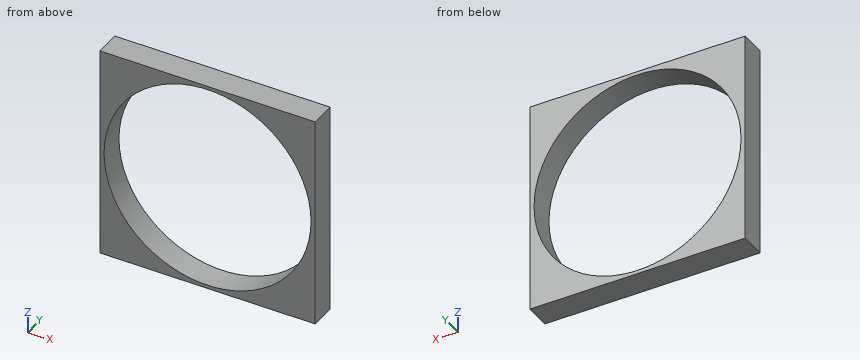
from build123d import *

# Parameters (mm, degrees)
F0_W     = 211.11551
F0_H     = 209.385068
F0_R     = 101.410764
F1_DEPTH = 25.4
F2_DEPTH = 25.4


with BuildPart() as f1:
    # F0 (on Front) → F1 (new body)
    with BuildSketch(Plane.XZ):
        Rectangle(F0_W, F0_H)
        Circle(F0_R, mode=Mode.SUBTRACT)
    extrude(amount=F1_DEPTH)

    # F0 (on Front) → F2 (join)
    with BuildSketch(Plane.XZ):
        Rectangle(F0_W, F0_H)
        Circle(F0_R, mode=Mode.SUBTRACT)
    extrude(amount=F2_DEPTH)


solid = f1.part
Design review of the part built by this model. Coordinates are the model's own, in mm. Give positions to 0.01 mm unless a question says otherwise; leave off trailing zeros. Order: outer loops, then holes, each group sorted by start corner. A loop starts at its lowest first (then second) coordinate and runs counter-clockwise, first axis right, second up. Notation, with made-up numbers: (18, 73.5) - (68, 73.5) arc R25 cw to (68, 102.5) - close; hole circle Ø7 at (82, 71). An arc over 180 degrees is marked (long way). Write item = value, one per line. Start each with the question number.
Q1. We need section A-A on x = 0. State the section outline as (y, z) points, plus the area to 3 significant figures.
Q2. We need section C-C on y = -3.5. State the section outline as (x, z) points.
Q3. We need section B-B on z = 0. State the section outline as (x, y) points, plus the area to 3 significant figures.
Q4. To check wall thickness, follow L1, parallel to Z at x = 0, y = -15.25; L2, parallel to Z at x = 64.5, y = -2.5; L3, parallel to X at y = -22.25, z = 63. State the ranges of each line that lie inside material, in increasing order. Write a range as from..to.
Working result:
q1.outline = (-25.4, -104.69) - (0, -104.69) - (0, -101.41) - (-25.4, -101.41) - close; (-25.4, 101.41) - (0, 101.41) - (0, 104.69) - (-25.4, 104.69) - close
q1.area = 167 mm²
q2.outline = (-105.56, -104.69) - (105.56, -104.69) - (105.56, 104.69) - (-105.56, 104.69) - close; hole circle Ø202.82 at (0, 0)
q3.outline = (-105.56, -25.4) - (-101.41, -25.4) - (-101.41, 0) - (-105.56, 0) - close; (101.41, -25.4) - (105.56, -25.4) - (105.56, 0) - (101.41, 0) - close
q3.area = 211 mm²
q4.L1 = -104.69..-101.41, 101.41..104.69
q4.L2 = -104.69..-78.26, 78.26..104.69
q4.L3 = -105.56..-79.47, 79.47..105.56
